Can you work these out from the model? Positions are in its coordinate system, mm. Face numbers are marked on the shaded views. Round coordinates to 2 decimals unless told otherwise and drop trailing zeros. Write each loop counter-clockwise with the first axis right and the second up, starting at its lowest first coordinate (ties: lowest second). Pieces come first, ordered by that corner, then holes. Notation, with made-up numbers: (43, 67) -> (61, 67) arc R23 ccw to (61, 82) -> close; hole circle Ø6 at (84, 78). An arc over 180 degrees is marked (long way). Use CSV: the item, a comma, the result in double quotes.
```python
from build123d import *

# Parameters (mm, degrees)
CROQUIS1_W              = 40
CROQUIS1_H              = 67
SALIENTE_EXTRUIR1_DEPTH = 20
REDONDEO1_R             = 2
VACIADO1_START          = -18
VACIADO1_OUTLINE_W      = 65
VACIADO1_OUTLINE_H      = 16
VACIADO1_DEPTH          = 36
CROQUIS2_W              = 40
CROQUIS2_H              = 4
CORTAR_EXTRUIR1_DEPTH   = 15


# Read off the part's stored shape, not the designer's step: Vaciado1
with BuildPart() as part:
    # Croquis1 → Saliente-Extruir1 (new body)
    with BuildSketch(Plane.XY):
        Rectangle(CROQUIS1_W, CROQUIS1_H)
    extrude(amount=SALIENTE_EXTRUIR1_DEPTH)

    # Redondeo1
    redondeo1_edges = [part.edges().sort_by_distance(p)[0] for p in [
        (-20, 0, 20),
        (0, -33.5, 20),
        (20, 0, 20),
        (0, -33.5, 0),
        (-20, 0, 0),
        (20, 0, 0),
        (20, -33.5, 10),
        (-20, -33.5, 10),
    ]]
    fillet(redondeo1_edges, radius=REDONDEO1_R)

    # Vaciado1 outline → Vaciado1 (cut)
    with BuildSketch(Plane.YZ.offset(VACIADO1_START)):
        with Locations((-1, 10)):
            Rectangle(VACIADO1_OUTLINE_W, VACIADO1_OUTLINE_H)
    extrude(amount=VACIADO1_DEPTH, mode=Mode.SUBTRACT)

    # Croquis2 → Cortar-Extruir1 (cut)
    with BuildSketch(Plane(origin=(0, 33.5, 0), x_dir=(1, 0, 0), z_dir=(0, 1, 0))):
        with Locations((0, -10)):
            Rectangle(CROQUIS2_W, CROQUIS2_H)
    extrude(amount=-CORTAR_EXTRUIR1_DEPTH, mode=Mode.SUBTRACT)


solid = part.part
```
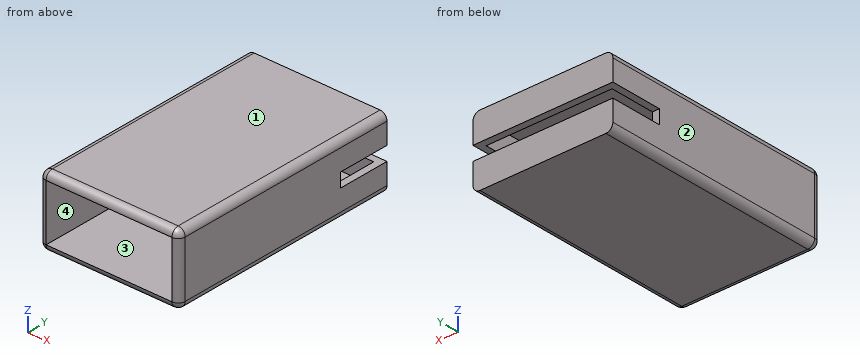
Q1. If we mould it in two halves opening along X, with no side actions, what happens to the marked faces 1, 2, 3 and 4? For each: released by +X, released by -X, zero draft, split by the parting line, or undercut.
Resolved:
face 1,"zero draft"
face 2,"released by -X"
face 3,"undercut"
face 4,"undercut"
Q2. Suppose I cut it at B-B (y = -19.5). Write out the boundary of the cut face in (x, z), and give its area (3 significant figures).
Resolved:
outline,"(-20, 2) arc R2 ccw to (-18, 0) -> (18, 0) arc R2 ccw to (20, 2) -> (20, 18) arc R2 ccw to (18, 20) -> (-18, 20) arc R2 ccw to (-20, 18) -> close; hole (-18, 2) -> (18, 2) -> (18, 18) -> (-18, 18) -> close"
area,"221 mm^2"
Q3. Suppose I cut it at C-C (z = 16.25). Write out the boundary of the cut face in (x, y).
Resolved:
outline,"(-20, -31.5) arc R2 ccw to (-18, -33.5) -> (-18, 31.5) -> (18, 31.5) -> (18, -33.5) arc R2 ccw to (20, -31.5) -> (20, 33.5) -> (-20, 33.5) -> close"
Q4. Suppose I cut it at A-A (x = -16.5). Write out the boundary of the cut face in (y, z).
Resolved:
outline,"(-33.5, 2) arc R2 ccw to (-31.5, 0) -> (33.5, 0) -> (33.5, 8) -> (31.5, 8) -> (31.5, 2) -> close; (-33.5, 18) -> (31.5, 18) -> (31.5, 12) -> (33.5, 12) -> (33.5, 20) -> (-31.5, 20) arc R2 ccw to start"
Q5. Will these pins go through, and if not, where does the flat tip stop? P1, Ø1.6, axis at x = 18.5, z = 9, coming from the +Y side; P2, Ø10, axis at x = 7.5, z = 9.5, coming from the -Y side; P3, Ø4, axis at y = 23, z = 11.5, coming from the -X side; P4, Ø1, axis at x = -7, z = 9.5, coming from the +Y side.
Resolved:
P1,"stops at y = 18.5"
P2,"stops at y = 31.5"
P3,"stops at x = -20"
P4,"passes through"
Q6. Please list where these lines run through material, in increasing order: probe 1 along Z at (x, y) = (11, -25.5); probe 2 along X at (y, z) = (1.5, 3.5); probe 3 along Y at (x, z) = (-7.5, 7).
Resolved:
probe 1,"z = 0 to 2, 18 to 20"
probe 2,"x = -20 to -18, 18 to 20"
probe 3,"y = 31.5 to 33.5"
